```python
from build123d import *

# Parameters (mm, degrees)
SKETCH2_R           = 1.6
BOSS_EXTRUDE1_DEPTH = 5
SKETCH3_R           = 10
BOSS_EXTRUDE2_DEPTH = 3
BOSS_EXTRUDE2_TAPER = 60
CUT_EXTRUDE1_REACH  = 63.555
SKETCH4_R           = 1.6
SKETCH5_R           = 3.5
CUT_EXTRUDE2_DEPTH  = 3
SKETCH6_R           = 3.2
CUT_EXTRUDE3_DEPTH  = 3


with BuildPart() as part:
    # Sketch2 → Boss-Extrude1 (new body)
    with BuildSketch(Plane(origin=(0, 0, 0), x_dir=(1, 0, 0), z_dir=(0, 1, 0))):
        with BuildLine():
            Line((-25, 0), (-25, 37))
            ThreePointArc((-25, 37), (-24.121320344, 39.121320344), (-22, 40))
            Line((-22, 40), (-10.477922061, 40))
            ThreePointArc((-10.477922061, 40), (-8.947188332, 39.69551813), (-7.649494937, 38.828427125))
            Line((-7.649494937, 38.828427125), (2.214466094, 28.964466094))
            ThreePointArc((2.214466094, 28.964466094), (5.75, 27.5), (9.285533906, 28.964466094))
            Line((9.285533906, 28.964466094), (19.149494937, 38.828427125))
            ThreePointArc((19.149494937, 38.828427125), (20.447188332, 39.69551813), (21.977922061, 40))
            Line((21.977922061, 40), (22, 40))
            ThreePointArc((22, 40), (24.121320344, 39.121320344), (25, 37))
            Line((25, 37), (25, 3))
            ThreePointArc((25, 3), (25.878679656, 0.878679656), (28, 0))
            Line((28, 0), (32, 0))
            ThreePointArc((32, 0), (34.121320344, 0.878679656), (35, 3))
            Line((35, 3), (35, 46))
            ThreePointArc((35, 46), (33.828427125, 48.828427125), (31, 50))
            Line((31, 50), (-31, 50))
            ThreePointArc((-31, 50), (-33.828427125, 48.828427125), (-35, 46))
            Line((-35, 46), (-35, 0))
            Line((-35, 0), (-35, -1))
            ThreePointArc((-35, -1), (-34.121320344, -3.121320344), (-32, -4))
            Line((-32, -4), (-28, -4))
            ThreePointArc((-28, -4), (-25.878679656, -3.121320344), (-25, -1))
            Line((-25, -1), (-25, 0))
        make_face()
        with Locations(Location((5.75, 32.5, 0), (0, 0, 270))):
            Circle(SKETCH2_R, mode=Mode.SUBTRACT)
        with BuildLine():
            Line((32.45, 45.5), (32.45, 35.5))
            ThreePointArc((32.45, 35.5), (30.75, 33.8), (29.05, 35.5))
            Line((29.05, 35.5), (29.05, 45.5))
            ThreePointArc((29.05, 45.5), (30.75, 47.2), (32.45, 45.5))
        make_face(mode=Mode.SUBTRACT)
        with BuildLine():
            Line((32.45, 13.5), (32.45, 3.5))
            ThreePointArc((32.45, 3.5), (30.75, 1.8), (29.05, 3.5))
            Line((29.05, 3.5), (29.05, 13.5))
            ThreePointArc((29.05, 13.5), (30.75, 15.2), (32.45, 13.5))
        make_face(mode=Mode.SUBTRACT)
        with BuildLine():
            Line((-29.05, 45.5), (-29.05, 35.5))
            ThreePointArc((-29.05, 35.5), (-30.75, 33.8), (-32.45, 35.5))
            Line((-32.45, 35.5), (-32.45, 45.5))
            ThreePointArc((-32.45, 45.5), (-30.75, 47.2), (-29.05, 45.5))
        make_face(mode=Mode.SUBTRACT)
        with BuildLine():
            Line((-29.05, 10.5), (-29.05, 0.5))
            ThreePointArc((-29.05, 0.5), (-30.75, -1.2), (-32.45, 0.5))
            Line((-32.45, 0.5), (-32.45, 10.5))
            ThreePointArc((-32.45, 10.5), (-30.75, 12.2), (-29.05, 10.5))
        make_face(mode=Mode.SUBTRACT)
    extrude(amount=BOSS_EXTRUDE1_DEPTH)

    # Sketch3 → Boss-Extrude2 (add)
    with BuildSketch(Plane(origin=(0, 5, 0), x_dir=(1, 0, 0), z_dir=(0, 1, 0))):
        with Locations((5.75, 32.5)):
            Circle(SKETCH3_R)
    extrude(amount=BOSS_EXTRUDE2_DEPTH, taper=BOSS_EXTRUDE2_TAPER)

    # Sketch4 → Cut-Extrude1 (cut, up to next)
    with BuildSketch(Plane.XZ, mode=Mode.PRIVATE) as cut_extrude1_sk1:
        with Locations(Location((5.75, -32.5, 0), (0, 0, 90))):
            Circle(SKETCH4_R)
    cut_extrude1_tool1 = extrude(cut_extrude1_sk1.sketch, amount=-CUT_EXTRUDE1_REACH, mode=Mode.PRIVATE) & part.part
    # Sketch4 → Cut-Extrude1 (cut, up to next)
    with BuildSketch(Plane.XZ, mode=Mode.PRIVATE) as cut_extrude1_sk2:
        with Locations(Location((5.75, -44.5, 0), (0, 0, 270))):
            Circle(SKETCH4_R)
    cut_extrude1_tool2 = extrude(cut_extrude1_sk2.sketch, amount=-CUT_EXTRUDE1_REACH, mode=Mode.PRIVATE) & part.part
    # Sketch4 → Cut-Extrude1 (cut, up to next)
    with BuildSketch(Plane.XZ, mode=Mode.PRIVATE) as cut_extrude1_sk3:
        with BuildLine():
            Line((-3.909258263, -35.088190451), (2.214466094, -28.964466094))
            ThreePointArc((2.214466094, -28.964466094), (5.75, -27.5), (9.285533906, -28.964466094))
            Line((9.285533906, -28.964466094), (15.409258263, -35.088190451))
            ThreePointArc((15.409258263, -35.088190451), (5.75, -22.5), (-3.909258263, -35.088190451))
        make_face()
    cut_extrude1_tool3 = extrude(cut_extrude1_sk3.sketch, amount=-CUT_EXTRUDE1_REACH, mode=Mode.PRIVATE) & part.part
    add(cut_extrude1_tool1.solids().sort_by_distance((5.75, 0, -32.5))[0], mode=Mode.SUBTRACT)
    add(cut_extrude1_tool2.solids().sort_by_distance((5.75, 0, -44.5))[0], mode=Mode.SUBTRACT)
    add(cut_extrude1_tool3.solids().sort_by_distance((12.514498, 0, -31.859226))[0], mode=Mode.SUBTRACT)

    # Sketch5 → Cut-Extrude2 (cut)
    with BuildSketch(Plane.XZ):
        with Locations(Location((5.75, -32.5, 0), (0, 0, 270))):
            Circle(SKETCH5_R)
    extrude(amount=-CUT_EXTRUDE2_DEPTH, mode=Mode.SUBTRACT)

    # Sketch6 → Cut-Extrude3 (cut)
    with BuildSketch(Plane(origin=(0, 5, 0), x_dir=(1, 0, 0), z_dir=(0, 1, 0))):
        with Locations((5.75, 44.5)):
            Circle(SKETCH6_R)
    extrude(amount=CUT_EXTRUDE3_DEPTH, mode=Mode.SUBTRACT)


solid = part.part
```
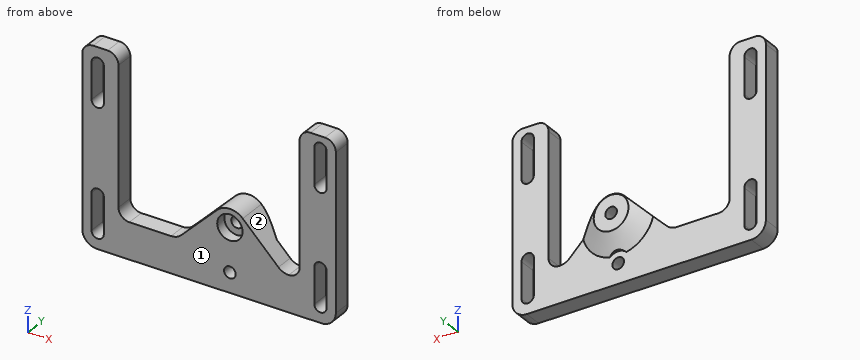
Model file for the job. Use its own axes, mm. Face numbers are marked on the shaded views. A direction names the side the tool comes from. Give positions to 0.01 mm unless a question says otherwise; leave off trailing zeros. Loops run counter-clockwise (first coordinate to the right, second up) from the corner with the lowest first, then second, coordinate; pieces in that order, holes last. Notation, with made-up numbers: (-17, 60) -> (3, 60) arc R32 cw to (3, 86) -> close; hole circle Ø5 at (0, 47.5). An arc over 180 degrees is marked (long way). Write each question's results on one line, items separated by ' | '.
(1) Probe line 1 along X through (y, z) = (1.65, -44.5); line 2 along X through (y, z) = (3.75, -42.5); line 3 along X through (y, z) = (1.25, -24.5). List the from-to ranges inside material, lowest first.
Geometry results:
line 1: x = -35 to -32.45, -29.05 to 4.15, 7.35 to 29.05, 32.45 to 35 | line 2: x = -35 to -32.45, -29.05 to 29.05, 32.45 to 35 | line 3: x = -35 to -25, 25 to 35
(2) Cut at A-A on x = 5.75. List the corners of the cut face in (y, z).
Geometry results:
outline: (0, -50) -> (5, -50) -> (5, -46.1) -> (0, -46.1) -> close; (0, -42.9) -> (5, -42.9) -> (5, -41.3) -> (5.69, -41.3) -> (8, -37.3) -> (8, -34.1) -> (3, -34.1) -> (3, -36) -> (0, -36) -> close; (0, -29) -> (3, -29) -> (3, -30.9) -> (8, -30.9) -> (8, -27.7) -> (7.89, -27.5) -> (0, -27.5) -> close
(3) Cut at B-B on z = -44.5. List the corners of the cut face in (x, y).
Geometry results:
outline: (-35, 0) -> (-32.45, 0) -> (-32.45, 5) -> (-35, 5) -> close; (-29.05, 0) -> (4.15, 0) -> (4.15, 5) -> (-29.05, 5) -> close; (7.35, 0) -> (29.05, 0) -> (29.05, 5) -> (7.35, 5) -> close; (32.45, 0) -> (35, 0) -> (35, 5) -> (32.45, 5) -> close
(4) Tool access for the marked faces 1 and 2: list every direction of +Z, -Z, +X, -X, +Y, -Y with a clear straight run to the whole face (end or side of a thin tool).
Geometry results:
face 1: +Z, -Z, +X, -X, -Y | face 2: +Z, +Y, -Y
(5) Cut at D-D on y = 1.5. Give the number of separate pieces and of enclosed holes in the cut face, and give its area (3 significant figures).
Geometry results:
separate pieces: 1 | enclosed holes: 6 | area: 1,520 mm²
(6) Flat gauge pins, fed straight in: pin 1 Ø2.5 at (x, y) = (-18.5, 3.5) entering from +Z; pin 2 Ø4 at (x, y) = (8, 3.5) entering from +Z; pin 3 Ø12 at (x, z) = (-20, -5) entering from +Y. Where does each tip first touch, or does it go through?
Geometry results:
pin 1: stops at z = -40 | pin 2: stops at z = -27.51 | pin 3: stops at y = 5
(7) Cut at C-C on z = -17. List the corners of the cut face in (x, y).
Geometry results:
outline: (-35, 0) -> (-25, 0) -> (-25, 5) -> (-35, 5) -> close; (25, 0) -> (35, 0) -> (35, 5) -> (25, 5) -> close
